Source: CAD feature listing. Evaluate the final solid. Frame: model axes, mm. Face numbers are marked on the shaded views. A direction names the side the tool comes from. Give positions to 0.01 mm unless a question says otherwise; leave off trailing zeros. Order: outer loops, then holes, each group sorted by start corner. A loop starts at its lowest first (then second) coordinate and runs counter-clockwise, first axis right, second up.
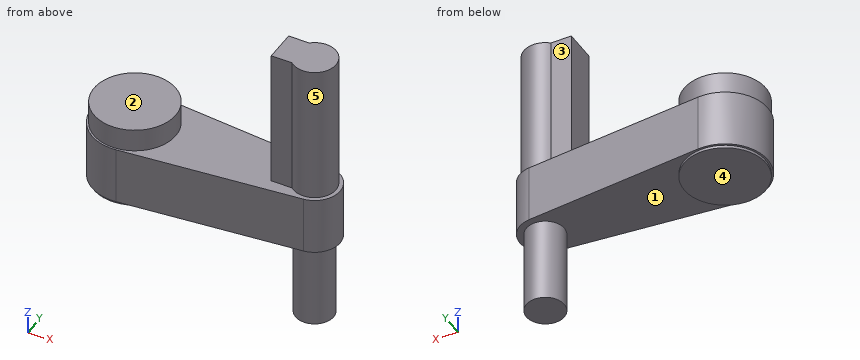
Autodesk Inventor part; units mm, degrees
ref_plane "YZ Plane" through (0, 0, 0) normal (1, 0, 0) x (0, 1, 0)
ref_plane "XZ Plane" through (0, 0, 0) normal (0, 1, 0) x (-1, 0, 0)
ref_plane "XY Plane" through (0, 0, 0) normal (0, 0, 1) x (1, 0, 0)
sketch "Sketch1" plane through (0, 0, 0) normal (0, 0, 1) x (1, 0, 0)
  circle A0 centre (0, 0) radius 85
  dimension "d0" = 170
extrude "Extrusion1" add sketch "Sketch1" along normal blind 6
sketch "Sketch2" plane through (0, 0, 6) normal (0, 0, 1) x (1, 0, 0)
  circle A0 centre (0, 0) radius 89 construction
  circle A1 centre (375, 0) radius 53 construction
  line L0 (8.544, 88.5889) -> (380.088, 52.7552)
  line L1 (8.544, -88.5889) -> (380.088, -52.7552)
  arc A2 (8.544, 88.5889) -> (8.544, -88.5889) centre (0, 0) ccw
  arc A3 (380.088, -52.7552) -> (380.088, 52.7552) centre (375, 0) ccw
  dimension "d3" = 178
  dimension "d4" = 106
  dimension "d5" = 375
extrude "Extrusion2" add sketch "Sketch2" along normal blind 121
sketch "Sketch3" plane through (0, 0, 127) normal (0, 0, 1) x (1, 0, 0)
  circle A0 centre (0, 0) radius 85
  dimension "d8" = 170
extrude "Extrusion3" add sketch "Sketch3" along normal blind 48
sketch "Sketch4" plane through (0, 0, 127) normal (0, 0, 1) x (1, 0, 0)
  arc A0 (380.088, -52.7552) -> (380.088, 52.7552) centre (375, 0) ccw construction
  circle A1 centre (375, 0) radius 44.5 construction
  line L0 (302.5, 33.375) -> (302.5, -33.375)
  line L1 (302.5, 33.375) -> (345.566, 33.375)
  line L2 (302.5, -33.375) -> (345.566, -33.375)
  arc A2 (345.566, -33.375) -> (345.566, 33.375) centre (375, 0) ccw
  point P0 (0, 0)
  point P1 (302.5, 0)
  dimension "d11" = 89
  dimension "d12" = 66.75
  dimension "d13" = 72.5
extrude "Extrusion4" add sketch "Sketch4" along normal blind 292
sketch "Sketch5" plane through (0, 0, 6) normal (0, 0, -1) x (-1, 0, 0)
  arc A0 (-380.088, 52.7552) -> (-380.088, -52.7552) centre (-375, 0) ccw construction
  circle A1 centre (-375, 0) radius 39.5
  point P0 (0, 0)
  dimension "d16" = 79
extrude "Extrusion5" add sketch "Sketch5" along normal blind 177.92
properties part number "2"
1) Section query C-C, the plane z = 260. Return the cut outline in (x, y) (3 decimals), and give its area (3 significant figures).
Report:
outline: (302.5, -33.375) - (345.566, -33.375) arc R44.5 ccw (long way) to (345.566, 33.375) - (302.5, 33.375) - close
area: 8,400 mm2
2) Material intervals for L1, parallel to Z at x = 314, y = -57; L2, parallel to Z at x = 9.5, y = 26; L3, parallel to Y at x = 375, z = -93, sorted ascending.
Report:
L1: z = 6 to 127
L2: z = 0 to 175
L3: y = -39.5 to 39.5
3) Reachability of the marked faces 1, 2, 3, 4 and 5 from +Z, -Z, +X, -X, +Y, -Y: full face, straight path, thin tool, end or side. Return the list, or none.
Report:
face 1: -Z
face 2: +Z, -X, +Y, -Y
face 3: +Z, +Y
face 4: -Z, -X, +Y, -Y
face 5: +Z
4) Pin query (flat end, axial travel): pin 1 (12 mm diameter, centred on y = -28, z = 94, fed in from -X); pin 2 (12 mm diameter, centred on x = 293, y = -39.5, fed in from +Z); pin 3 (13 mm diameter, centred on x = 326, z = 243, fed in from -Y) (3 decimals). Return the tip coordinate at first contact, or that it passes through.
Report:
pin 1: stops at x = -86.24
pin 2: stops at z = 127
pin 3: stops at y = -33.375
5) Section query A-A, the plane y = 0. Return the cut outline in (x, z), and give its area (3 significant figures).
Report:
outline: (-89, 6) - (-85, 6) - (-85, 0) - (85, 0) - (85, 6) - (335.5, 6) - (335.5, -171.92) - (414.5, -171.92) - (414.5, 6) - (428, 6) - (428, 127) - (419.5, 127) - (419.5, 419) - (302.5, 419) - (302.5, 127) - (85, 127) - (85, 175) - (-85, 175) - (-85, 127) - (-89, 127) - close
area: 120,000 mm2
6) Section query B-B, the plane x = 0. Return the cut outline in (y, z).
Report:
outline: (-89, 6) - (-85, 6) - (-85, 0) - (85, 0) - (85, 6) - (89, 6) - (89, 127) - (85, 127) - (85, 175) - (-85, 175) - (-85, 127) - (-89, 127) - close
7) Section query D-D, the plane y = -61. Return the cut outline in (x, z).
Report:
outline: (-64.81, 6) - (-59.19, 6) - (-59.19, 0) - (59.19, 0) - (59.19, 6) - (294.6, 6) - (294.6, 127) - (59.19, 127) - (59.19, 175) - (-59.19, 175) - (-59.19, 127) - (-64.81, 127) - close
